Study the drawing (mm; zero at the part's minimum x, y, z) and answer. Give positions to 0.01 mm unless a question says otherwise; leave off trailing zeros. Write each loop counter-clockwise with the first axis right and the second up, starting at its lowest first coordinate (ties: lowest second). Pieces come first, ordered by that corner, then holes. Notation, with made-up numbers: (24.5, -24.75) - (66.5, -24.75) arc R28 ccw to (66.5, -3.75) - close; hole circle Ø3 at (62.5, -25). An arc over 180 degrees is marked (long way). Answer as CSV lines item,"result".
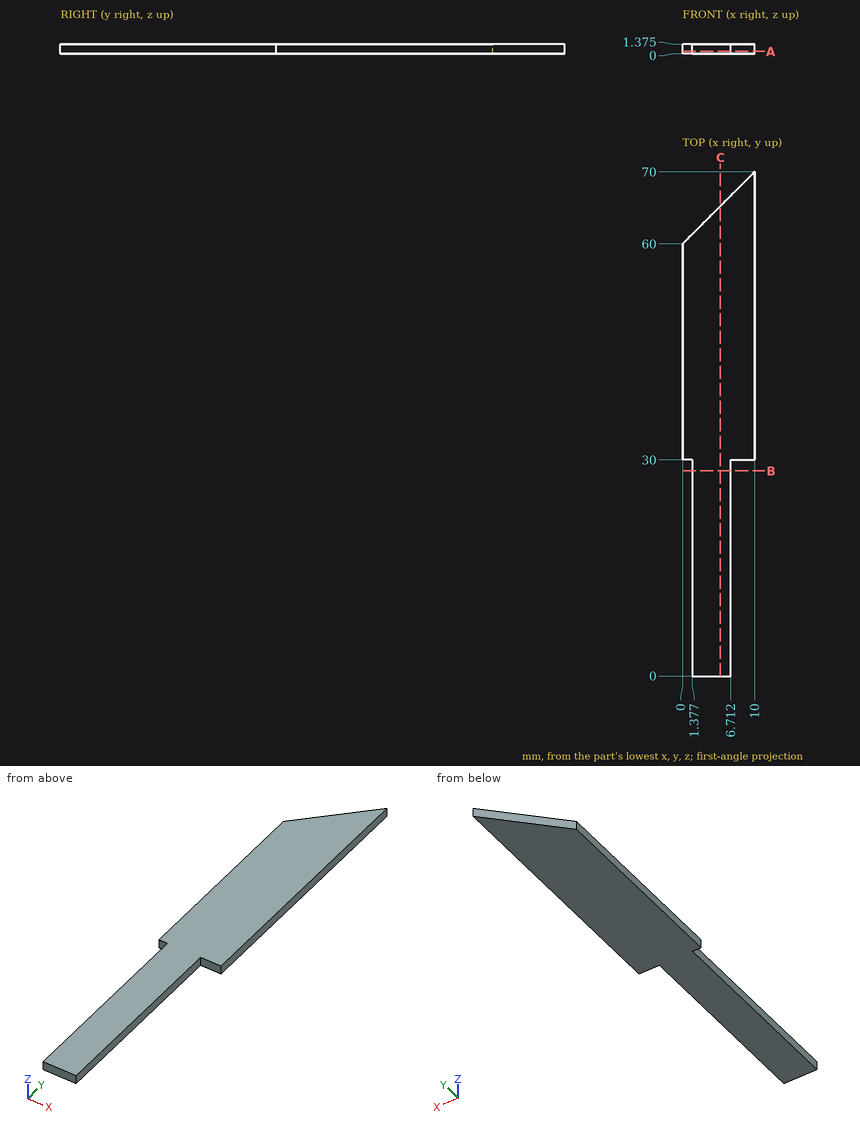
(1) A cutting plane is placed at B-B (y = 28.5). Write down the section's boundary in (x, z) (3 decimals), and give its area (3 significant figures).
Worked out:
outline,"(1.377, 0) - (6.712, 0) - (6.712, 1.375) - (1.377, 1.375) - close"
area,"7.34 mm^2"
(2) A cutting plane is placed at A-A (z = 0.35). Write down the section's boundary in (x, y).
Worked out:
outline,"(0, 30) - (1.38, 30) - (1.38, 0) - (6.71, 0) - (6.71, 30) - (10, 30) - (10, 70) - (0, 60) - close"
(3) Find the intervals of material crossed by L1, parallel to X at y = 16, z = 0.3; L2, parallel to Y at x = 8, z = 0.95; L3, parallel to Y at x = 6.25, z = 0.4, in increasing order.
Worked out:
L1,"x = 1.38 to 6.71"
L2,"y = 30 to 68"
L3,"y = 0 to 66.25"
(4) A cutting plane is placed at C-C (x = 5.25). Write down the section's boundary in (y, z) (3 decimals).
Worked out:
outline,"(0, 0) - (65.25, 0) - (65.25, 1.375) - (0, 1.375) - close"
